```python
from build123d import *

# Parameters (mm, degrees)
SHELL1_T = -1


with BuildPart() as part:
    # Sketch2 → Revolve1 (revolve)
    with BuildSketch(Plane.XY, mode=Mode.PRIVATE) as revolve1_sk:
        with BuildLine():
            Line((15, 0), (15, 2))
            Line((15, 2), (17, 2))
            Line((17, 2), (14.292893219, 4.707106781))
            ThreePointArc((14.292893219, 4.707106781), (13.96846987, 4.923879533), (13.585786438, 5))
            Line((13.585786438, 5), (0, 5))
            Line((0, 5), (0, 0))
            Line((0, 0), (15, 0))
        make_face()
    revolve(revolve1_sk.sketch.rotate(Axis((0, 5, 0), (0, -1, 0)), 90), axis=Axis((0, 5, 0), (0, -1, 0)))

    # Shell1
    shell1_openings = [part.faces().sort_by_distance(p)[0] for p in [
        (0, 0, 0),
    ]]
    offset(amount=SHELL1_T, openings=shell1_openings, kind=Kind.INTERSECTION)


solid = part.part
```
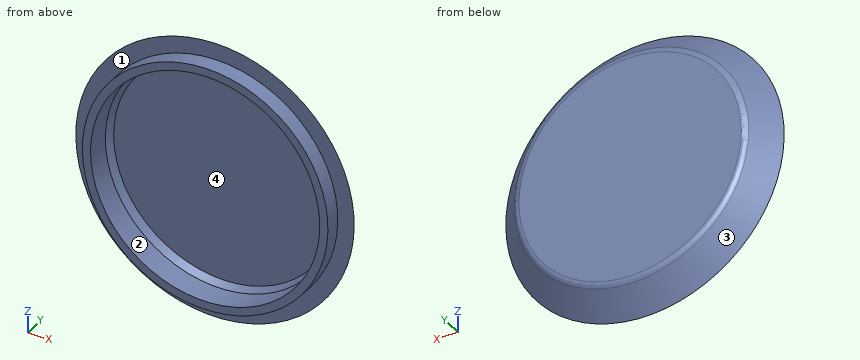
Check sheet for the modelled part. Datum: model origin and axes. Units: mm. Face numbers are marked on the shaded views. Round coordinates to 2 decimals unless told otherwise and drop trailing zeros. Order: outer loops, then holes, each group sorted by start corner. A loop starts at its lowest first (then second) coordinate and runs counter-clockwise, first axis right, second up. Notation, with made-up numbers: (48.5, 32.5) -> (101.5, 32.5) arc R23 ccw to (101.5, 67.5) -> close; hole circle Ø5 at (-12, -40). An arc over 180 degrees is marked (long way). One line per item, written item: value. Start each with the question number.
Q1. Cross-section at A-A (z = 0). Record the boundary of the cut face in (x, y).
Q2. Cross-section at D-D (y = 3.6). Record the boundary of the cut face in (x, z).
Q3. Mould release check, pull along Z, two halves, no side actions. Record for the marked faces 1, 2, 3 and 4: pulls with the +Z half, pulls with the -Z half, needs draft (parallel to the pull), parting line crosses it, or undercut.
Q4. Cross-section at B-B (x = 0). Record the boundary of the cut face in (y, z), and give its area (3 significant figures).
Q5. Thickness scan on line 1 (X direction, y = 1.4, z = 0); line 2 (Y direction, x = 6, z = 8); line 3 (Z direction, x = 2.5, y = 2.15). Record the ranges inside material, lowest first.
Q6. Gauge pin test, flat ends, axial feed: pin 1 Ø1.5 at (x, z) = (12, -3) entering from -Y; pin 2 Ø1.5 at (x, z) = (-13, -11) entering from -Y. Record the tip position at first contact, or that the pin passes through.
Q7. Cross-section at C-C (y = 0.5). Record the boundary of the cut face in (x, z), and give its area (3 significant figures).
Completed:
1. outline: (-17, 2) -> (-15, 2) -> (-15, 0) -> (-14, 0) -> (-14, 3) -> (-14.59, 3) -> (-13.59, 4) -> (13.59, 4) -> (14.59, 3) -> (14, 3) -> (14, 0) -> (15, 0) -> (15, 2) -> (17, 2) -> (14.29, 4.71) arc R1 ccw to (13.59, 5) -> (-13.59, 5) arc R1 ccw to (-14.29, 4.71) -> close
2. outline: circle Ø30.8 at (0, 0); hole circle Ø27.97 at (0, 0)
3. face 1: needs draft
3. face 2: undercut
3. face 3: parting line crosses it
3. face 4: undercut
4. outline: (0, -15) -> (2, -15) -> (2, -17) -> (4.71, -14.29) arc R1 ccw to (5, -13.59) -> (5, 13.59) arc R1 ccw to (4.71, 14.29) -> (2, 17) -> (2, 15) -> (0, 15) -> (0, 14) -> (3, 14) -> (3, 14.59) -> (4, 13.59) -> (4, -13.59) -> (3, -14.59) -> (3, -14) -> (0, -14) -> close
4. area: 40.8 mm²
5. line 1: x = -15 to -14, 14 to 15
5. line 2: y = 4 to 5
5. line 3: z = -16.66 to -13.77, 13.77 to 16.66
6. pin 1: stops at y = 4
6. pin 2: stops at y = 2
7. outline: circle Ø30 at (0, 0); hole circle Ø28 at (0, 0)
7. area: 91.1 mm²
